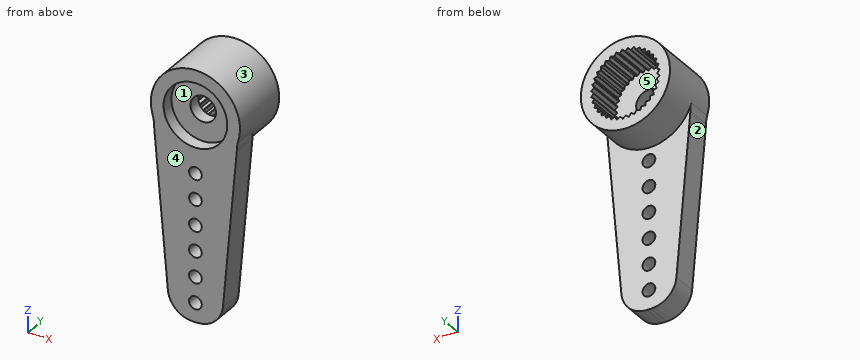
from build123d import *

# Parameters (mm, degrees)
BOSS_EXTRUDE1_DEPTH      = 2
FILLET1_R                = 2
BOSS_EXTRUDE2_DEPTH      = 3
BOSS_EXTRUDE2_DEPTH_BACK = 2
SKETCH2_R                = 3.5
SKETCH3_R                = 2.5
CUT_EXTRUDE1_DEPTH       = 1
SKETCH4_R                = 1
CUT_EXTRUDE2_DEPTH       = 17.8597153
CUT_EXTRUDE3_START       = -3
SKETCH5_R                = 2.5
CUT_EXTRUDE3_DEPTH       = 3
CUT_EXTRUDE4_DEPTH       = 3
CIRPATTERN1_COUNT        = 36
SKETCH9_R                = 0.5
CUT_EXTRUDE5_DEPTH       = 18.12454379
LPATTERN1_COUNT          = 6
LPATTERN1_PITCH          = 2
FILLET3_R                = 2


with BuildPart() as part:
    # Sketch1 → Boss-Extrude1 (new body)
    with BuildSketch(Plane(origin=(0, 0, 0), x_dir=(1, 0, 0), z_dir=(0, 1, 0))):
        Polygon((-3.25, 0), (-3.25, 1.75), (-2, 16), (2, 16), (3.25, 1.75), (3.25, 0), align=None)
    extrude(amount=BOSS_EXTRUDE1_DEPTH)

    # Fillet1
    fillet1_edges = [part.edges().sort_by_distance(p)[0] for p in [
        (-2, 1, -16),
        (2, 1, -16),
    ]]
    fillet(fillet1_edges, radius=FILLET1_R)

    # Sketch2 → Boss-Extrude2 (add, two sides: drawn at the far end of the back side and taken through both)
    with BuildSketch(Plane(origin=(0, 2, 0), x_dir=(1, 0, 0), z_dir=(0, 1, 0)).offset(-BOSS_EXTRUDE2_DEPTH_BACK)):
        with Locations(Location((0, 0, 0), (0, 0, 270))):
            Circle(SKETCH2_R)
    extrude(amount=BOSS_EXTRUDE2_DEPTH + BOSS_EXTRUDE2_DEPTH_BACK)

    # Sketch3 → Cut-Extrude1 (cut)
    with BuildSketch(Plane(origin=(0, 0, 0), x_dir=(-1, 0, 0), z_dir=(0, -1, 0))):
        with Locations(Location((0, 0, 0), (0, 0, 90))):
            Circle(SKETCH3_R)
    extrude(amount=-CUT_EXTRUDE1_DEPTH, mode=Mode.SUBTRACT)

    # Sketch4 → Cut-Extrude2 (cut, through all)
    with BuildSketch(Plane(origin=(0, 1, 0), x_dir=(-1, 0, 0), z_dir=(0, -1, 0))):
        with Locations(Location((0, 0, 0), (0, 0, 90))):
            Circle(SKETCH4_R)
    extrude(amount=-CUT_EXTRUDE2_DEPTH, mode=Mode.SUBTRACT)

    # Sketch5 → Cut-Extrude3 (cut)
    with BuildSketch(Plane(origin=(0, 5, 0), x_dir=(1, 0, 0), z_dir=(0, 1, 0)).offset(CUT_EXTRUDE3_START)):
        with Locations(Location((0, 0, 0), (0, 0, 90))):
            Circle(SKETCH5_R)
    extrude(amount=CUT_EXTRUDE3_DEPTH, mode=Mode.SUBTRACT)

    # Sketch6 → Cut-Extrude4 (cut)
    with BuildSketch(Plane(origin=(0, 5, 0), x_dir=(1, 0, 0), z_dir=(0, 1, 0))):
        Polygon((-2.5, 0), (-2.691676801, 0.211839558), (-2.469220851, 0.391086163), align=None)
    cut_extrude4 = extrude(amount=-CUT_EXTRUDE4_DEPTH, mode=Mode.SUBTRACT)

    # CirPattern1: Cut-Extrude4 ×36 about axis
    cirpattern1_axis = Axis((0, 0, 0), (0, 1, 0))
    for i in range(1, CIRPATTERN1_COUNT):
        add(cut_extrude4.rotate(cirpattern1_axis, i * 360 / CIRPATTERN1_COUNT), mode=Mode.SUBTRACT)

    # Sketch9 → Cut-Extrude5 (cut, through all)
    with BuildSketch(Plane(origin=(0, 0, 0), x_dir=(-1, 0, 0), z_dir=(0, -1, 0))):
        with Locations(Location((0, 14.5, 0), (0, 0, 90))):
            Circle(SKETCH9_R)
    cut_extrude5 = extrude(amount=-CUT_EXTRUDE5_DEPTH, mode=Mode.SUBTRACT)

    # LPattern1: Cut-Extrude5 ×6
    with Locations(*[(0, 0, i * LPATTERN1_PITCH) for i in range(1, LPATTERN1_COUNT)]):
        add(cut_extrude5, mode=Mode.SUBTRACT)

    # Fillet3
    # the kernel refuses this fillet: 2 mm, written as the material it adds along each edge
    with BuildSketch(Plane(origin=(-3.25, 0, -1.299038106), x_dir=(0, 0, -1), z_dir=(0, 1, 0))) as fillet3_piece_1:
        with BuildLine():
            CenterArc((0.340321525, 2), FILLET3_R, 252.658557197, 17.341442803)
            ThreePointArc((-0.25580925, 0.090909091), (-0.127022856, 0.047935757), (0, 0))
            Line((0, 0), (0.340321525, 0))
        make_face()
    extrude(amount=2)
    with BuildSketch(Plane(origin=(3.25, 0, -1.299038106), x_dir=(0.3348614999479688, 0, 0.9422673590083636), z_dir=(0, 1, 0))) as fillet3_piece_2:
        with BuildLine():
            CenterArc((0.349049135, 1.998495294), FILLET3_R, 250.435883949, 17.341442803)
            Line((-0.320673865, 0.113960576), (0, 0))
            ThreePointArc((0, 0), (0.13574133, 0.002633235), (0.271482661, 0))
        make_face()
    extrude(amount=2)
    # the kernel refuses this fillet: 2 mm, written as the material it takes off along each edge
    with BuildSketch(Plane(origin=(3.25, -0.218878004, -1.75), x_dir=(0, 0, 1), z_dir=(0, 1, 0)), Plane(origin=(-3.25, -0.218878004, -1.75), x_dir=(0.08738374771484407, 0, -0.9961747239492218), z_dir=(0, 1, 0))) as fillet3_2_piece_1:
        with BuildLine():
            CenterArc((FILLET3_R * 0.043775600736, -FILLET3_R), FILLET3_R, 90, 5.013113755)
            Line((-FILLET3_R * 0.0436081469789, -FILLET3_R * 0.00382527605078), (0, 0))
            Line((0, 0), (FILLET3_R * 0.043775600736, 0))
        make_face()
    extrude(amount=2.437756007, mode=Mode.SUBTRACT)


solid = part.part
Design review of the part built by this model. Coordinates are the model's own, in mm. Face numbers are marked on the shaded views. A direction names the side the tool comes from. Round coordinates to 2 decimals unless told otherwise and drop trailing zeros. Write each loop counter-clockwise with the first axis right and the second up, starting at its lowest first coordinate (ties: lowest second). Pieces come first, ordered by that corner, then holes. Notation, with made-up numbers: M 32.5,57.5 L 53.5,57.5 A26 cw 53.5,87.5 Z; hole C 46,55.25 d10. An arc over 180 degrees is marked long. One line per item, written item: value. Start each with the question number.
1. Clearance check with flat-ended pins moving along their axes: P1, Ø3, axis at x = 0, z = 0, coming from the -Y side; P2, Ø3, axis at y = 2.5, z = -12, coming from the +X side. State where each tip first meets the part, or that it passes through.
2. To check wall thickness, follow probe 1 along X at (y, z) = (0.55, -4.5); probe 2 along X at (y, z) = (1.4, -14.5); probe 3 along Y at (x, z) = (3, -2.25). State the ranges of each line that lie inside material, in increasing order. Write a range as from..to.
3. Take a section at A-A on y = 0.55. State how many separate pieces and enclosed holes the cut face has, then the cut area to 3 significant figures.
4. Draft analysis for pull direction Z (two halves, no side actions). For the marked faces 3, 4 and 5, state which applies: pulls with the +Z half, pulls with the -Z half, needs draft (parallel to the pull), parting line crosses it, or undercut.
5. For the marked faces 1 and 2, list the 3-axis set-ups (+Z, -Z, +X, -X, +Y, -Y) from which the entire face can be reached by the end or side of a thin tool; tool diameter is ignored.
6. Take a section at C-C on z = -12.5. State the section outline as (x, y) points.
7. Take a section at B-B on z = -8.5. State the section outline as (x, y) points, then the cut area to 3 significant figures.
Computed:
1. P1: stops at y = 1
1. P2: stops at x = 2.47
2. probe 1: x = -3.01..-0.5, 0.5..3.01
2. probe 2: x = -2.1..-0.5, 0.5..2.1
2. probe 3: y = 0..2
3. separate pieces: 1
3. enclosed holes: 7
3. area: 80.1 mm²
4. face 3: parting line crosses it
4. face 4: needs draft
4. face 5: undercut
5. face 1: -Y
5. face 2: -Z, -X, +Y, -Y
6. outline: M -2.31,0 L -0.5,0 L -0.5,2 L -2.31,2 Z; M 0.5,0 L 2.31,0 L 2.31,2 L 0.5,2 Z
7. outline: M -2.66,0 L -0.5,0 L -0.5,2 L -2.66,2 Z; M 0.5,0 L 2.66,0 L 2.66,2 L 0.5,2 Z
7. area: 8.63 mm²
